Answer from the drawing. Dimensions are ordinates in mm from the lowest x, y and z of the part. Give positions to 0.01 mm unless a question says otherwise; leave off trailing zeros. Loops run counter-clockwise (first coordinate to the right, second up) from the corner with the lowest first, then second, coordinate; pieces in that order, holes last. Notation, with made-up numbers: (0, 81.5) -> (33, 81.5) arc R23 cw to (33, 109.5) -> close; hole circle Ø6 at (34, 59.5). An arc over 180 degrees is marked (long way). Return JSON: item names as keys, results as strings. Group by question number.
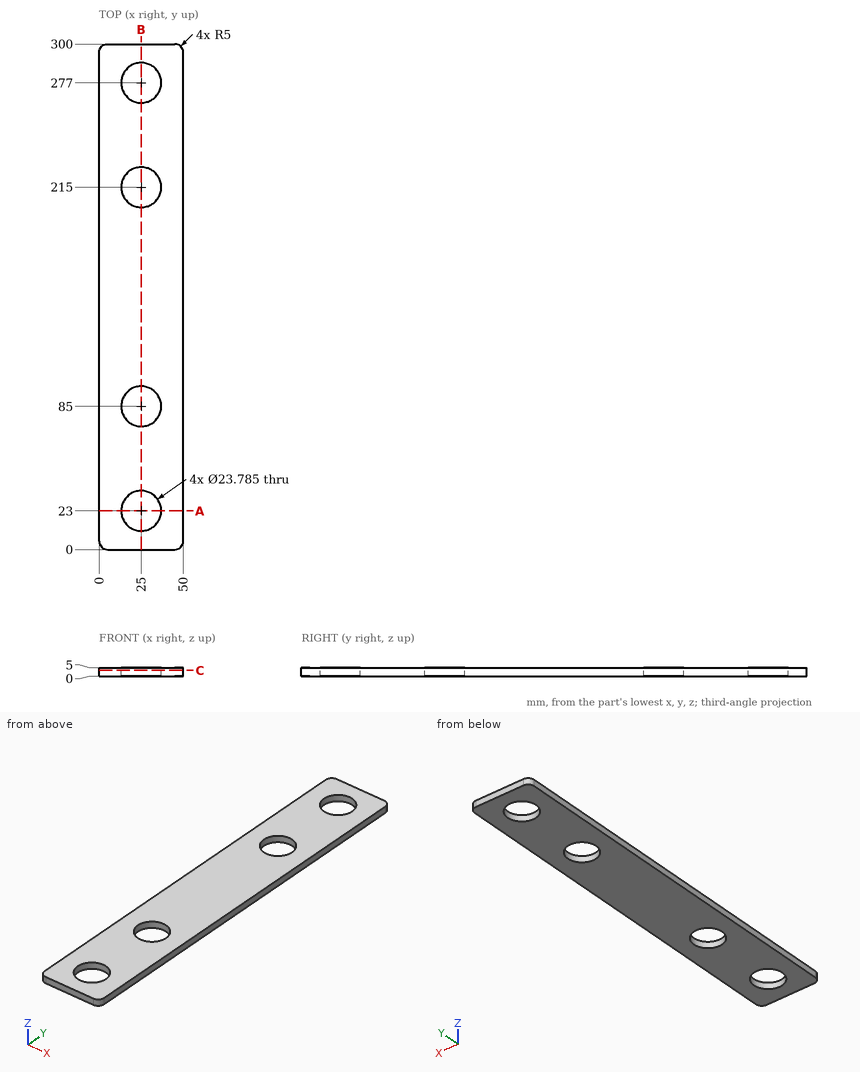
1. Flat-ended cylindrical pins translate along their axes: pin 1 Ø14.5 at (x, y) = (25, 277) entering from +Z; pin 2 Ø1 at (x, y) = (42, 159) entering from -Z. Find the tip coordinate at first contact, or state that the pin passes through.
2. Section B-B on x = 25 is taken. Determine the outline of the cut face in (y, z), then the cut area to 3 significant figures.
3. Section C-C on z = 3.4 is taken. Determine the outline of the cut face in (x, y) (1 decimal).
4. Straight lines are drawn through the part: line 1 (Y direction, x = 26, z = 4.6); line 2 (Y direction, x = 25, z = 2.3); line 3 (X direction, y = 276, z = 1.15). For each, find the intervals that lie inside material, in ascending order. Write a range as from..to.
5. Section A-A on y = 23 is taken. Determine the outline of the cut face in (x, z).
Completed:
{
 "1": {"pin 1": "passes through", "pin 2": "stops at z = 0"},
 "2": {"outline": "(0, 0) -> (11.11, 0) -> (11.11, 5) -> (0, 5) -> close; (34.89, 0) -> (73.11, 0) -> (73.11, 5) -> (34.89, 5) -> close; (96.89, 0) -> (203.11, 0) -> (203.11, 5) -> (96.89, 5) -> close; (226.89, 0) -> (265.11, 0) -> (265.11, 5) -> (226.89, 5) -> close; (288.89, 0) -> (300, 0) -> (300, 5) -> (288.89, 5) -> close", "area": "1,020 mm²"},
 "3": {"outline": "(0, 5) arc R5 ccw to (5, 0) -> (45, 0) arc R5 ccw to (50, 5) -> (50, 295) arc R5 ccw to (45, 300) -> (5, 300) arc R5 ccw to (0, 295) -> close; hole circle Ø23.8 at (25, 23); hole circle Ø23.8 at (25, 85); hole circle Ø23.8 at (25, 215); hole circle Ø23.8 at (25, 277)"},
 "4": {"line 1": "y = 0..11.15, 34.85..73.15, 96.85..203.15, 226.85..265.15, 288.85..300", "line 2": "y = 0..11.11, 34.89..73.11, 96.89..203.11, 226.89..265.11, 288.89..300", "line 3": "x = 0..13.15, 36.85..50"},
 "5": {"outline": "(0, 0) -> (13.11, 0) -> (13.11, 5) -> (0, 5) -> close; (36.89, 0) -> (50, 0) -> (50, 5) -> (36.89, 5) -> close"}
}
